Autodesk Inventor part; units mm, degrees
ref_plane "YZ Plane" through (0, 0, 0) normal (1, 0, 0) x (0, 1, 0)
ref_plane "XZ Plane" through (0, 0, 0) normal (0, 1, 0) x (-1, 0, 0)
ref_plane "XY Plane" through (0, 0, 0) normal (0, 0, 1) x (1, 0, 0)
sketch "Skizze1" plane through (0, 0, 0) normal (0, 0, 1) x (1, 0, 0)
  line L0 (-7.2, 0) -> (43.2, 0)
  line L1 (0, -6.6) -> (0, 39.6)
  line L2 (0, 0) -> (36, 0)
  line L3 (36, 0) -> (36, 33)
  line L4 (36, 33) -> (0, 33)
  line L5 (0, 33) -> (0, 0)
  dimension "d0" = 36
  dimension "d1" = 33
extrude "Extrusion1" add sketch "Skizze1" along normal blind 3
sketch "Skizze2" plane through (0, 0, 3) normal (0, 0, 1) x (1, 0, 0)
  line L0 (0, 0) -> (36, 0)
  line L1 (36, 0) -> (36, 33)
  line L2 (36, 33) -> (0, 33)
  line L3 (0, 33) -> (0, 0)
  line L4 (5, 28) -> (31, 28)
  line L5 (31, 28) -> (31, 5)
  line L6 (31, 5) -> (5, 5)
  line L7 (5, 5) -> (5, 28)
  line L8 (18, 33) -> (18, 0)
  line L9 (36, 16.5) -> (0, 16.5)
  dimension "d4" = 26
  dimension "d5" = 23
hole "Bohrung1" at (31, 28, 3) at (5, 5, 3) direction (0, 0, -1) diameter 3.4 end through all countersink diameter 6.9 countersink angle 90
properties part number "13_1087_014"
The listing builds one solid part. Answer for the finished solid, in the listing's coordinates (mm). Give positions to 0.01 mm unless a question says otherwise; leave off trailing zeros. Write each loop counter-clockwise with the first axis right and the second up, starting at its lowest first coordinate (ties: lowest second). Pieces come first, ordered by that corner, then holes.
1) Given P1, Ø1, axis at y = 16, z = 1.5, coming from the -X side; P2, Ø3, axis at x = 31, y = 28, coming from the +Z side, each flat-ended and moving along its own axis, determine where each tip first touches the part or whether it passes through.
2) Section C-C (x = 31) is taken. Write down the section's boundary in (y, z).
3) Section B-B (y = 28) is taken. Write down the section's boundary in (x, z), and give its area (3 significant figures).
4) For a pull along X with two mould halves and no side action, classify faces 1 (the face through (4.307, 3.329, 1.359)), 2 (the face through (18, 17, 0)), 3 (the face through (36, 16, 1)) as pulls with the +X half, pulls with the -X half, needs draft (parallel to the pull), parting line crosses it, or undercut.
5) Find the intervals of material crossed by L1, parallel to X at y = 28, z = 0.65; L2, parallel to Y at x = 5, z = 1.05; L3, parallel to Y at x = 31, z = 0.65, in increasing order.
6) Section A-A (z = 0.45) is taken. Write down the section's boundary in (x, y).
Response:
1. P1: stops at x = 0
1. P2: passes through
2. outline: (0, 0) - (26.3, 0) - (26.3, 1.25) - (24.55, 3) - (0, 3) - close; (29.7, 0) - (33, 0) - (33, 3) - (31.45, 3) - (29.7, 1.25) - close
3. outline: (0, 0) - (29.3, 0) - (29.3, 1.25) - (27.55, 3) - (0, 3) - close; (32.7, 0) - (36, 0) - (36, 3) - (34.45, 3) - (32.7, 1.25) - close
3. area: 94.7 mm2
4. face 1: undercut
4. face 2: needs draft
4. face 3: pulls with the +X half
5. L1: x = 0 to 29.3, 32.7 to 36
5. L2: y = 0 to 3.3, 6.7 to 33
5. L3: y = 0 to 26.3, 29.7 to 33
6. outline: (0, 0) - (36, 0) - (36, 33) - (0, 33) - close; hole circle Ø3.4 at (5, 5); hole circle Ø3.4 at (31, 28)
